```python
from build123d import *

# Parameters (mm, degrees)
F0_W        = 200
F0_H        = 340
F1_DEPTH    = 35
F2_W        = 15
F2_H        = 130
F3_DEPTH    = 0.5
F4_R        = 25
F5_T1_DEPTH = 357.7701999818
F6_R        = 10
F8_DEPTH    = 97.478


# Not quite as in the source:
# - a fillet or chamfer that OpenCascade refuses, or shapes differently, is made with other operations: its cross-section is extruded or revolved along the edge and cut away or added


with BuildPart() as f1:
    # F0 (on Top) → F1 (new body)
    with BuildSketch(Plane.XY):
        Rectangle(F0_W, F0_H)
    extrude(amount=F1_DEPTH)

    # F2 (on face) → F3 (cut)
    with BuildSketch(Plane(origin=(0, 0, 0), x_dir=(1, 0, 0), z_dir=(0, 0, -1))):
        with Locations((-50, 95)):
            Rectangle(F2_W, F2_H)
        with Locations((50, 95)):
            Rectangle(F2_W, F2_H)
        with Locations((-50, -95)):
            Rectangle(F2_W, F2_H)
        with Locations((50, -95)):
            Rectangle(F2_W, F2_H)
    extrude(amount=-F3_DEPTH, mode=Mode.SUBTRACT)

    # F4
    f4_edges = [f1.edges().sort_by_distance(p)[0] for p in [
        (100, -170, 17.5),
        (-100, -170, 17.5),
        (100, 170, 17.5),
        (-100, 170, 17.5),
    ]]
    fillet(f4_edges, radius=F4_R)

    # F5: chamfer of 40 x 10 on 2 edges, made by hand

    # F5_s2 → F5_t1 (cut)
    with BuildSketch(Plane.YZ.offset(-178.8850999909)):
        Polygon((-160, 0), (-170, 40), (-170, 0), align=None)
        Polygon((170, 40), (160, 0), (170, 0), align=None)
    extrude(amount=F5_T1_DEPTH, mode=Mode.SUBTRACT)

    # F6
    f6_edges = [f1.edges().sort_by_distance(p)[0] for p in [
        (0, -168.75, 35),
    ]]
    fillet(f6_edges, radius=F6_R)

    # F7 (on Right) → F8 (join, symmetric)
    with BuildSketch(Plane.YZ):
        with BuildLine():
            Line((-155.942235936, 35), (-100.942235936, 35))
            Line((-100.942235936, 35), (-100.942235936, 90))
            ThreePointArc((-100.942235936, 90), (-139.8331089012, 73.8908729653), (-155.942235936, 35))
        make_face()
        with BuildLine():
            ThreePointArc((-50.942235936, 85), (-86.2975749953, 70.3553390593), (-100.942235936, 35))
            Line((-100.942235936, 35), (-50.942235936, 35))
            Line((-50.942235936, 35), (-50.942235936, 85))
        make_face()
        with BuildLine():
            ThreePointArc((-5.942235936, 80), (-37.7620410894, 66.8198051534), (-50.942235936, 35))
            Line((-50.942235936, 35), (-5.942235936, 35))
            Line((-5.942235936, 35), (-5.942235936, 75))
            Line((-5.942235936, 75), (-5.942235936, 80))
        make_face()
        with BuildLine():
            ThreePointArc((159.057764064, 50), (148.4511623462, 45.6066017178), (144.057764064, 35))
            Line((144.057764064, 35), (159.057764064, 35))
            Line((159.057764064, 35), (159.057764064, 50))
        make_face()
        with BuildLine():
            ThreePointArc((34.057764064, 75), (5.7734928166, 63.2842712475), (-5.942235936, 35))
            Line((-5.942235936, 35), (34.057764064, 35))
            Line((34.057764064, 35), (34.057764064, 70))
            Line((34.057764064, 70), (34.057764064, 75))
        make_face()
        with BuildLine():
            ThreePointArc((69.057764064, 70), (44.3090267225, 59.7487373415), (34.057764064, 35))
            Line((34.057764064, 35), (69.057764064, 35))
            Line((69.057764064, 35), (69.057764064, 65))
            Line((69.057764064, 65), (69.057764064, 70))
        make_face()
        with BuildLine():
            ThreePointArc((99.057764064, 65), (77.8445606284, 56.2132034356), (69.057764064, 35))
            Line((69.057764064, 35), (99.057764064, 35))
            Line((99.057764064, 35), (99.057764064, 60))
            Line((99.057764064, 60), (99.057764064, 65))
        make_face()
        with BuildLine():
            ThreePointArc((124.057764064, 60), (106.3800945344, 52.6776695297), (99.057764064, 35))
            Line((99.057764064, 35), (124.057764064, 35))
            Line((124.057764064, 35), (124.057764064, 55))
            Line((124.057764064, 55), (124.057764064, 60))
        make_face()
        with BuildLine():
            ThreePointArc((144.057764064, 55), (129.9156284403, 49.1421356237), (124.057764064, 35))
            Line((124.057764064, 35), (144.057764064, 35))
            Line((144.057764064, 35), (144.057764064, 50))
            Line((144.057764064, 50), (144.057764064, 55))
        make_face()
    extrude(amount=F8_DEPTH, both=True)


solid = f1.part
```
CAD build for the part. Positions are in the model's coordinates, mm. A direction names the side the tool comes from. Round coordinates to 2 decimals unless told otherwise and drop trailing zeros. Order: outer loops, then holes, each group sorted by start corner. A loop starts at its lowest first (then second) coordinate and runs counter-clockwise, first axis right, second up. Notation, with made-up numbers: (30.25, -17) - (87.25, -17) arc R25 ccw to (87.25, 10) - close; hole circle Ø10 at (40.5, 6.5). An arc over 180 degrees is marked (long way). Answer in a Markdown table with one row per item. Add a question column.
(1) 3-axis set-ups, long thin cutter, end or side, ignore diameter. For faces 5 (the face through (-97.478, 153, 41)), 6 (the face through (-50, -96, 0.5)), 7 (the face through (97.478, 87, 47)), 8 (the face through (1.36, -139.4, 74.32)): which of +Z, -Z, +X, -X, +Y, -Y reach the whole face in a straight line?
(2) Band-saw the part on B-B on y = -109. List the corners of the cut face in (x, z).
(3) Band-saw the part on D-D on z = 9. List the corners of the cut face in (x, y).
(4) Band-saw the part on C-C on z = 42.5. Count the separate pieces of the cut face and the enclosed holes in it, and give its area (3 significant figures).
(5) Probe L1, parallel to Y at x = 74, z = 62; L2, parallel to Y at x = -9, z = 62.5; L3, parallel to Z at x = -23, y = -124. List the from-to ranges inside material, lowest first. Write a range as [from, to].
(6) Mould opens along Y. For faces 1 (the face through (1.36, -85.91, 70.74)), 2 (the face through (97.478, 136, 43)), 3 (the face through (1, 159.058, 42)), 4 (the face through (1.36, -163.75, 31.25)) say: +Y half, -Y half, draft (parallel to the pull), parting line (faces both ways), or undercut.
(7) Drop flat-ended pins along their axis: pin 1 Ø5 at (x, z) = (-25, 9.5) entering from +Y; pin 2 Ø4 at (x, z) = (-55.5, 28) entering from -Y; pin 3 Ø4 at (y, z) = (-6, 72.5) entering from -X; pin 4 Ø1.4 at (x, y) = (-96, 157.5) entering from -Z. Give the stop position or say it passes through.
(8) Band-saw the part on A-A on x = -35.5. List the corners of the cut face in (y, z), and give its area (3 significant figures).
Data:
| question | item | result |
|---|---|---|
| 1 | face 5 | +Z, -X, +Y, -Y |
| 1 | face 6 | -Z |
| 1 | face 7 | +Z, +X, +Y, -Y |
| 1 | face 8 | +Z, +X, -X, -Y |
| 2 | outline | (-100, 0) - (-57.5, 0) - (-57.5, 0.5) - (-42.5, 0.5) - (-42.5, 0) - (42.5, 0) - (42.5, 0.5) - (57.5, 0.5) - (57.5, 0) - (100, 0) - (100, 35) - (97.48, 35) - (97.48, 89.41) - (-97.48, 89.41) - (-97.48, 35) - (-100, 35) - close |
| 3 | outline | (-100, -145) arc R25 ccw to (-93.1, -162.25) - (93.1, -162.25) arc R25 ccw to (100, -145) - (100, 145) arc R25 ccw to (93.1, 162.25) - (-93.1, 162.25) arc R25 ccw to (-100, 145) - close |
| 4 | separate pieces | 9 |
| 4 | enclosed holes | 0 |
| 4 | area | 59,700 mm^2 |
| 5 | L1 | y = [-148.86, -100.94], [-93.03, -50.94], [-41.94, -5.94], [4.55, 34.06], [46.79, 69.06], [85.98, 99.06] |
| 5 | L2 | y = [-148.57, -100.94], [-92.7, -50.94], [-41.56, -5.94], [5.01, 34.06], [47.41, 69.06], [87.07, 99.06] |
| 5 | L3 | z = [0, 84.93] |
| 6 | face 1 | undercut |
| 6 | face 2 | draft |
| 6 | face 3 | +Y half |
| 6 | face 4 | -Y half |
| 7 | pin 1 | stops at y = 163 |
| 7 | pin 2 | stops at y = -165.89 |
| 7 | pin 3 | stops at x = -97.48 |
| 7 | pin 4 | stops at z = 0 |
| 8 | outline | (-165.64, 22.57) - (-160, 0) - (160, 0) - (168.75, 35) - (159.06, 35) - (159.06, 50) arc R15 ccw to (144.06, 35) - (144.06, 55) arc R20 ccw to (124.06, 35) - (124.06, 60) arc R25 ccw to (99.06, 35) - (99.06, 65) arc R30 ccw to (69.06, 35) - (69.06, 70) arc R35 ccw to (34.06, 35) - (34.06, 75) arc R40 ccw to (-5.94, 35) - (-5.94, 80) arc R45 ccw to (-50.94, 35) - (-50.94, 85) arc R50 ccw to (-100.94, 35) - (-100.94, 90) arc R55 ccw to (-155.94, 35) arc R10 ccw to start |
| 8 | area | 21,300 mm^2 |
